```python
from build123d import *

# Parameters (mm, degrees)
AUFSATZ_LINEAR_AUSTRAGEN1_DEPTH = 2


with BuildPart() as part:
    # Skizze2 → Aufsatz-Linear austragen1 (new body)
    with BuildSketch(Plane.XY):
        Polygon((0, 0), (95, 25.455173281), (95, 60), (85, 60), (55, 90), (95, 90), (95, 135), (0, 135), align=None)
        with BuildLine():
            Line((18, 111), (18, 59))
            ThreePointArc((18, 59), (14, 55), (10, 59))
            Line((10, 59), (10, 111))
            ThreePointArc((10, 111), (14, 115), (18, 111))
        make_face(mode=Mode.SUBTRACT)
    extrude(amount=AUFSATZ_LINEAR_AUSTRAGEN1_DEPTH)


solid = part.part
```
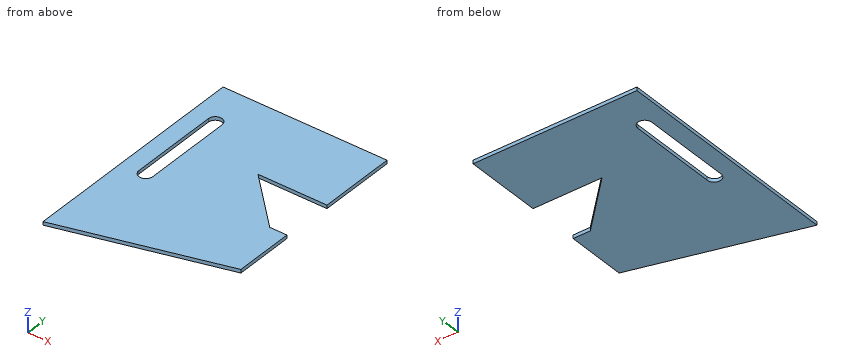
Can you work these out from the model? Positions are in its coordinate system, mm. Give positions to 0.01 mm unless a question says otherwise; leave off trailing zeros. Loops run counter-clockwise (first coordinate to the right, second up) from the corner with the lowest first, then second, coordinate; pieces in that order, holes last. Notation, with made-up numbers: M 65,-16.5 L 95,-16.5 A23 ccw 95,13.5 Z; hole C 73.25,12 d6. An arc over 180 degrees is marked long. Answer in a Markdown table with one row per item.
1. Suppose I cut it at C-C on x = 87. Write out the boundary of the cut face in (y, z).
Taken from the geometry:
| item | result |
|---|---|
| outline | M 23.31,0 L 60,0 L 60,2 L 23.31,2 Z; M 90,0 L 135,0 L 135,2 L 90,2 Z |
2. If I drill on line 1 along X through (y, z) = (93, 1.7); line 2 along Y through (x, z) = (71, 1.85); line 3 along X through (y, z) = (63, 1.05), over which ranges is the centre line in solid material (lowest first)?
Taken from the geometry:
| item | result |
|---|---|
| line 1 | x = 0 to 10, 18 to 95 |
| line 2 | y = 19.02 to 74, 90 to 135 |
| line 3 | x = 0 to 10, 18 to 82 |
3. Suppose I cut it at D-D on y = 14. Write out the boundary of the cut face in (x, z).
Taken from the geometry:
| item | result |
|---|---|
| outline | M 0,0 L 52.25,0 L 52.25,2 L 0,2 Z |
4. Suppose I cut it at A-A on y = 62.5. Write out the boundary of the cut face in (x, z).
Taken from the geometry:
| item | result |
|---|---|
| outline | M 0,0 L 10,0 L 10,2 L 0,2 Z; M 18,0 L 82.5,0 L 82.5,2 L 18,2 Z |
5. For pin 1 Ø1 at (y, z) = (85, 1) entering from +X; pin 2 Ø12 at (x, y) = (78, 32) entering from -Z; pin 3 Ø0.6 at (x, z) = (84, 1) entering from -Y, each with a flat end and sliding along its axis, tell me the tip position at first contact or that it passes through.
Taken from the geometry:
| item | result |
|---|---|
| pin 1 | stops at x = 60.5 |
| pin 2 | stops at z = 0 |
| pin 3 | stops at y = 22.43 |
6. Suppose I cut it at B-B on z = 1.55. Write out the boundary of the cut face in (x, y), plus the area to 3 significant figures.
Taken from the geometry:
| item | result |
|---|---|
| outline | M 0,0 L 95,25.46 L 95,60 L 85,60 L 55,90 L 95,90 L 95,135 L 0,135 Z; hole M 10,59 A4 ccw 18,59 L 18,111 A4 ccw 10,111 Z |
| area | 10,400 mm² |
